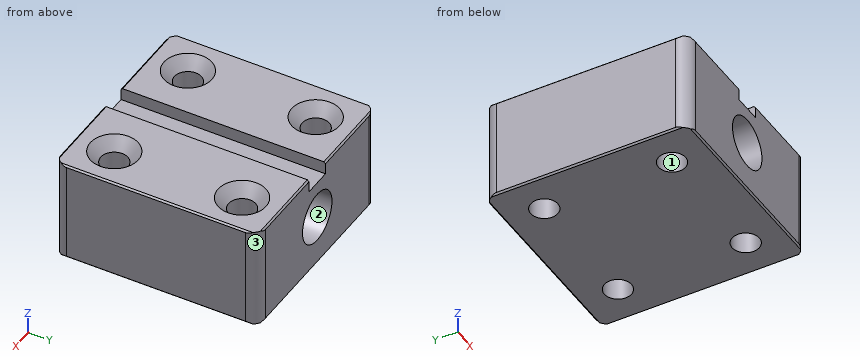
from build123d import *

# Parameters (mm, degrees)
F1_DEPTH       = 50.8
F3_D           = 13.49248
F3_CSINK_D     = 23.8252
F3_CSINK_ANGLE = 82
F4_SIZE        = 0.8128
F5_T1_DEPTH    = 80.9244
F7_D           = 25.4


# Not quite as in the source:
# - a fillet or chamfer that OpenCascade refuses, or shapes differently, is made with other operations: its cross-section is extruded or revolved along the edge and cut away or added


with BuildPart() as f1:
    # F0 (on Front) → F1 (new body, symmetric)
    with BuildSketch(Plane.XZ):
        Polygon((-7.0944838226, 25.4), (-50.8, 25.4), (-50.8, -25.4), (50.8, -25.4), (50.8, 25.4), (7.0944838226, 25.4), (7.0944838226, 19.05), (0, 19.05), (-7.0944838226, 19.05), align=None)
    extrude(amount=F1_DEPTH, both=True)

    # F3 (through all)
    with Locations(Plane.XY.offset(25.4)):
        with Locations((-31.75, 31.75), (31.75, 31.75), (31.75, -31.75), (-31.75, -31.75)):
            CounterSinkHole(F3_D / 2, F3_CSINK_D / 2, counter_sink_angle=F3_CSINK_ANGLE)

    # F4
    f4_edges = [f1.edges().sort_by_distance(p)[0] for p in [
        (-50.8, 0, 25.4),
        (50.8, 0, 25.4),
        (0, -50.8, -25.4),
        (-50.8, 0, -25.4),
        (0, 50.8, -25.4),
        (50.8, 0, -25.4),
        (-28.947242, -50.8, 25.4),
        (28.947242, -50.8, 25.4),
        (28.947242, 50.8, 25.4),
        (-28.947242, 50.8, 25.4),
    ]]
    chamfer(f4_edges, length=F4_SIZE)

    # F5: fillet of radius 6.35 on 4 edges, made by hand

    # F5_s2 → F5_t1 (cut)
    with BuildSketch(Plane.XY.offset(-40.4622)):
        with BuildLine():
            ThreePointArc((-44.45, -50.8), (-48.9401280605, -48.9401280605), (-50.8, -44.45))
            Line((-50.8, -44.45), (-50.8, -50.8))
            Line((-50.8, -50.8), (-44.45, -50.8))
        make_face()
        with BuildLine():
            ThreePointArc((44.45, -50.8), (48.9401280605, -48.9401280605), (50.8, -44.45))
            Line((50.8, -44.45), (50.8, -50.8))
            Line((50.8, -50.8), (44.45, -50.8))
        make_face()
        with BuildLine():
            ThreePointArc((44.45, 50.8), (48.9401280605, 48.9401280605), (50.8, 44.45))
            Line((50.8, 44.45), (50.8, 50.8))
            Line((50.8, 50.8), (44.45, 50.8))
        make_face()
        with BuildLine():
            ThreePointArc((-44.45, 50.8), (-48.9401280605, 48.9401280605), (-50.8, 44.45))
            Line((-50.8, 44.45), (-50.8, 50.8))
            Line((-50.8, 50.8), (-44.45, 50.8))
        make_face()
    extrude(amount=F5_T1_DEPTH, mode=Mode.SUBTRACT)

    # F7 (through all)
    with Locations(Plane.XZ.offset(50.8)):
        with Locations((0, 0)):
            Hole(F7_D / 2)


solid = f1.part
The model under review builds one solid part; all positions refer to its coordinate system, in mm. Face numbers are marked on the shaded views. Coordinates: 2 decimals unless noted, no trailing zeros. Write each loop counter-clockwise with the first axis right and the second up, starting at its lowest first coordinate (ties: lowest second). Pieces come first, ordered by that corner, then holes. Notation, with made-up numbers: (-35.5, 81.5) -> (-30.5, 81.5) arc R14 ccw to (-30.5, 92.5) -> close; hole circle Ø5 at (76.25, -19.5). An arc over 180 degrees is marked (long way). Answer in a Markdown table with one row per item.
1. We need section C-C, the plane x = 0. State the section outline as (y, z) points, and give its area (3 significant figures).
Answers below:
| item | result |
|---|---|
| outline | (-50.8, -24.59) -> (-49.99, -25.4) -> (49.99, -25.4) -> (50.8, -24.59) -> (50.8, -12.7) -> (-50.8, -12.7) -> close; (-50.8, 12.7) -> (50.8, 12.7) -> (50.8, 19.05) -> (-50.8, 19.05) -> close |
| area | 1,930 mm^2 |
2. Clearance check with a flat-ended pin moving along its axis: pin 1 Ø7 at (x, y) = (2, 3.5) entering from +Z. State where the tip first meets the part, or that it passes through.
Answers below:
| item | result |
|---|---|
| pin 1 | stops at z = 19.05 |
3. We need section D-D, the plane x = 31.75. State the section outline as (y, z) points, and give its area (3 significant figures).
Answers below:
| item | result |
|---|---|
| outline | (-50.8, -24.59) -> (-49.99, -25.4) -> (-38.5, -25.4) -> (-38.5, 19.46) -> (-43.66, 25.4) -> (-49.99, 25.4) -> (-50.8, 24.59) -> close; (-25, -25.4) -> (25, -25.4) -> (25, 19.46) -> (19.84, 25.4) -> (-19.84, 25.4) -> (-25, 19.46) -> close; (38.5, -25.4) -> (49.99, -25.4) -> (50.8, -24.59) -> (50.8, 24.59) -> (49.99, 25.4) -> (43.66, 25.4) -> (38.5, 19.46) -> close |
| area | 3,730 mm^2 |
4. Draft analysis for pull direction Y (two halves, no side actions). For the marked faces 1, 2 and 3, state which applies: +Y half, -Y half, draft (parallel to the pull), parting line (faces both ways), or undercut.
Answers below:
| item | result |
|---|---|
| face 1 | undercut |
| face 2 | draft |
| face 3 | +Y half |
5. We need section B-B, the plane y = -31.75. State the section outline as (x, z) points, and give its area (3 significant figures).
Answers below:
| item | result |
|---|---|
| outline | (-50.8, -24.59) -> (-49.99, -25.4) -> (-38.5, -25.4) -> (-38.5, 19.46) -> (-43.66, 25.4) -> (-49.99, 25.4) -> (-50.8, 24.59) -> close; (-25, -25.4) -> (25, -25.4) -> (25, 19.46) -> (19.84, 25.4) -> (7.09, 25.4) -> (7.09, 19.05) -> (-7.09, 19.05) -> (-7.09, 25.4) -> (-19.84, 25.4) -> (-25, 19.46) -> close; (38.5, -25.4) -> (49.99, -25.4) -> (50.8, -24.59) -> (50.8, 24.59) -> (49.99, 25.4) -> (43.66, 25.4) -> (38.5, 19.46) -> close; hole circle Ø25.4 at (0, 0) |
| area | 3,130 mm^2 |
6. We need section A-A, the plane z = 0. State the section outline as (x, y) points, and give its area (3 significant figures).
Answers below:
| item | result |
|---|---|
| outline | (-50.8, -44.45) arc R6.35 ccw to (-44.45, -50.8) -> (-12.7, -50.8) -> (-12.7, 50.8) -> (-44.45, 50.8) arc R6.35 ccw to (-50.8, 44.45) -> close; (12.7, -50.8) -> (44.45, -50.8) arc R6.35 ccw to (50.8, -44.45) -> (50.8, 44.45) arc R6.35 ccw to (44.45, 50.8) -> (12.7, 50.8) -> close; hole circle Ø13.49 at (-31.75, -31.75); hole circle Ø13.49 at (-31.75, 31.75); hole circle Ø13.49 at (31.75, -31.75); hole circle Ø13.49 at (31.75, 31.75) |
| area | 7,140 mm^2 |
7. Wall thickness on probe 1 along Y at (x, z) = (31.75, -15); probe 2 along Z at (x, y) = (-0.5, -11); probe 3 along X at (y, z) = (-31, -15): over which ranges is each line inside the solid? List them lowest first. Write a range as [from, to].
Answers below:
| item | result |
|---|---|
| probe 1 | y = [-50.8, -38.5], [-25, 25], [38.5, 50.8] |
| probe 2 | z = [-25.4, -12.69], [12.69, 19.05] |
| probe 3 | x = [-50.8, -38.45], [-25.05, 25.05], [38.45, 50.8] |
